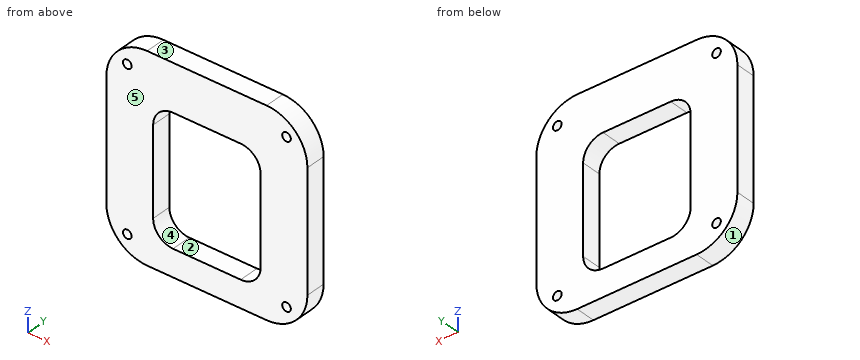
```python
from build123d import *

# Parameters (mm, degrees)
SKETCH_1_W          = 101
SKETCH_1_H          = 101
SKETCH_1_W_2        = 54
SKETCH_1_H_2        = 64
EXTRUDE_1_DEPTH     = 10
FILLET_1_R          = 20.5
FILLET_2_R          = 10
SKETCH_2_R          = 2.166
CUT_EXTRUDE_1_DEPTH = 73.114492302


with BuildPart() as part:
    # 草图1 → 凸台-拉伸1 (new body)
    with BuildSketch(Plane(origin=(0, 0, 0), x_dir=(1, 0, 0), z_dir=(0, 1, 0))):
        Rectangle(SKETCH_1_W, SKETCH_1_H)
        with Locations((0, 5)):
            Rectangle(SKETCH_1_W_2, SKETCH_1_H_2, mode=Mode.SUBTRACT)
    extrude(amount=EXTRUDE_1_DEPTH)

    # 圆角1
    fillet_1_edges = [part.edges().sort_by_distance(p)[0] for p in [
        (-50.5, 5, -50.5),
        (50.5, 5, -50.5),
        (50.5, 5, 50.5),
        (-50.5, 5, 50.5),
    ]]
    fillet(fillet_1_edges, radius=FILLET_1_R)

    # 圆角2
    fillet_2_edges = [part.edges().sort_by_distance(p)[0] for p in [
        (-27, 5, -37),
        (-27, 5, 27),
        (27, 5, 27),
        (27, 5, -37),
    ]]
    fillet(fillet_2_edges, radius=FILLET_2_R)

    # 草图2 → 切除-拉伸1 (cut, through all)
    with BuildSketch(Plane(origin=(0, 10, 0), x_dir=(1, 0, 0), z_dir=(0, 1, 0))):
        with Locations(Location((-40, 40, 0), (0, 0, 270))):
            Circle(SKETCH_2_R)
        with Locations(Location((40, 40, 0), (0, 0, 270))):
            Circle(SKETCH_2_R)
        with Locations(Location((-40, -40, 0), (0, 0, 270))):
            Circle(SKETCH_2_R)
        with Locations(Location((40, -40, 0), (0, 0, 270))):
            Circle(SKETCH_2_R)
    extrude(amount=-CUT_EXTRUDE_1_DEPTH, mode=Mode.SUBTRACT)


solid = part.part
```
Here's how the part is built. I have some questions about the finished solid (model axes, mm). Face numbers are marked on the shaded views. A direction names the side the tool comes from. Coordinates: 2 decimals unless noted, no trailing zeros. Write each loop counter-clockwise with the first axis right and the second up, starting at its lowest first coordinate (ties: lowest second). Pieces come first, ordered by that corner, then holes. Notation, with made-up numbers: (-38.5, 7) - (-21.5, 7) arc R16 ccw to (-21.5, 17) - close; hole circle Ø10 at (-30.75, 65.5). An arc over 180 degrees is marked (long way). One line per item, written item: value.
1) On a 3-axis mill with a long thin cutter (end or side, diameter ignored), from which of +Z, -Z, +X, -X, +Y, -Y can I reach the whole of each face in a straight line? I mean the marked faces 1 and 2. Say none if no direction works.
Model answer:
face 1: -Z, -X, +Y, -Y
face 2: +Y, -Y
2) We'd pull the mould along Z, two halves only. Please class the marked faces 3, 4 and 5: pulls with the +Z half, pulls with the -Z half, needs draft (parallel to the pull), parting line crosses it, or undercut.
Model answer:
face 3: pulls with the +Z half
face 4: undercut
face 5: needs draft
3) Suppose I cut it at C-C on x = 40. Write out the boundary of the cut face in (y, z).
Model answer:
outline: (0, -47.9) - (10, -47.9) - (10, -42.17) - (0, -42.17) - close; (0, -37.83) - (10, -37.83) - (10, 37.83) - (0, 37.83) - close; (0, 42.17) - (10, 42.17) - (10, 47.9) - (0, 47.9) - close
4) Suppose I cut it at B-B on x = -23. Write out the boundary of the cut face in (y, z).
Model answer:
outline: (0, -50.5) - (10, -50.5) - (10, -35) - (0, -35) - close; (0, 25) - (10, 25) - (10, 50.5) - (0, 50.5) - close
5) I'm going to push flat-ended pins straight in: P1, Ø3.5, axis at x = -40, z = -40, coming from the +Y side; P2, Ø1.5, axis at x = 36, y = 7.5, coming from the -Z side; P3, Ø7, axis at x = 40, z = 40, coming from the +Y side; P4, Ø2, axis at y = 4, z = 33.5, coming from the -X side. Where does each tip first touch, or does it pass through?
Model answer:
P1: passes through
P2: stops at z = -49.82
P3: stops at y = 10
P4: stops at x = -50.35
6) Suppose I cut it at D-D on z = 40. Write out the boundary of the cut face in (x, y), and give its area (3 significant figures).
Model answer:
outline: (-47.9, 0) - (-42.17, 0) - (-42.17, 10) - (-47.9, 10) - close; (-37.83, 0) - (37.83, 0) - (37.83, 10) - (-37.83, 10) - close; (42.17, 0) - (47.9, 0) - (47.9, 10) - (42.17, 10) - close
area: 871 mm²
7) Suppose I cut it at A-A on z = -11. Write out the boundary of the cut face in (x, y), and give its area (3 significant figures).
Model answer:
outline: (-50.5, 0) - (-27, 0) - (-27, 10) - (-50.5, 10) - close; (27, 0) - (50.5, 0) - (50.5, 10) - (27, 10) - close
area: 470 mm²
8) I need wall thicknesses on line 1 along X through (y, z) = (3.5, 2); line 2 along X through (y, z) = (5.5, 40); line 3 along Z through (x, y) = (-11, 3). Which ranges of each line are inside material? Lowest first, please.
Model answer:
line 1: x = -50.5 to -27, 27 to 50.5
line 2: x = -47.9 to -42.17, -37.83 to 37.83, 42.17 to 47.9
line 3: z = -50.5 to -37, 27 to 50.5
